Verification items for the finished model (mm, model axes). A direction names the side the tool comes from. Round coordinates to 2 decimals unless told otherwise and drop trailing zeros. Order: outer loops, then holes, each group sorted by start corner. A loop starts at its lowest first (then second) coordinate and runs counter-clockwise, first axis right, second up. Notation, with made-up numbers: (75, -33) -> (79, -33) arc R22 ccw to (79, 0) -> close; hole circle Ø9 at (-5.75, -23). An arc over 180 degrees is marked (long way). Put each result on its own line as item: value.
from build123d import *

# Parameters (mm, degrees)
BOSS_EXTRUDE1_DEPTH = 26
SKETCH3_R           = 2.25
CUT_EXTRUDE1_DEPTH  = 50.759421218
SKETCH2_R           = 2.5
CUT_EXTRUDE2_DEPTH  = 50.759421218
SKETCH4_R           = 5
CUT_EXTRUDE3_DEPTH  = 45.452221542
SKETCH5_R           = 4
CUT_EXTRUDE4_DEPTH  = 45.452221542
CHAMFER1_SIZE       = 3
FILLET2_R           = 4


with BuildPart() as part:
    # Sketch1 → Boss-Extrude1 (new body)
    with BuildSketch(Plane.XY):
        Polygon((0, 0), (10, 0), (30, 20), (30, 30), (0, 30), align=None)
    extrude(amount=BOSS_EXTRUDE1_DEPTH)

    # Sketch3 → Cut-Extrude1 (cut, through all)
    with BuildSketch(Plane(origin=(0, 30, 0), x_dir=(1, 0, 0), z_dir=(0, 1, 0))):
        with Locations(Location((20, -6, 0), (0, 0, 180))):
            Circle(SKETCH3_R)
    extrude(amount=-CUT_EXTRUDE1_DEPTH, mode=Mode.SUBTRACT)

    # Sketch2 → Cut-Extrude2 (cut, through all)
    with BuildSketch(Plane.ZY):
        with Locations(Location((18, 10, 0), (0, 0, 270))):
            Circle(SKETCH2_R)
    extrude(amount=-CUT_EXTRUDE2_DEPTH, mode=Mode.SUBTRACT)

    # Sketch4 → Cut-Extrude3 (cut, through all)
    with BuildSketch(Plane.ZY.offset(-10)):
        with Locations(Location((18, 10, 0), (0, 0, 270))):
            Circle(SKETCH4_R)
    extrude(amount=-CUT_EXTRUDE3_DEPTH, mode=Mode.SUBTRACT)

    # Sketch5 → Cut-Extrude4 (cut, through all)
    with BuildSketch(Plane(origin=(0, 20, 0), x_dir=(1, 0, 0), z_dir=(0, 1, 0))):
        with Locations(Location((20, -6, 0), (0, 0, 180))):
            Circle(SKETCH5_R)
    extrude(amount=-CUT_EXTRUDE4_DEPTH, mode=Mode.SUBTRACT)

    # Chamfer1
    # the kernel refuses this chamfer: 3 mm, written as the material it adds along each edge
    with BuildSketch(Plane(origin=(10, 10, 18), x_dir=(0, -1, 0), z_dir=(0, 0, -1))) as chamfer1_piece_1_section:
        Polygon((5, -CHAMFER1_SIZE), (5 - CHAMFER1_SIZE, 0), (5, 0), align=None)
    chamfer1_piece_1 = revolve(axis=Axis((10, 10, 18), (-1, 0, 0)), mode=Mode.PRIVATE)
    chamfer1_piece_1 = chamfer1_piece_1 - Plane(origin=(11.757355127, 10, 18), x_dir=(0, -1, 0), z_dir=(-1, 0, 0)) * Cylinder(2.5, 20, mode=Mode.PRIVATE)
    add(chamfer1_piece_1)

    # Fillet2
    fillet2_edges = [part.edges().sort_by_distance(p)[0] for p in [
        (30, 20, 13),
        (10, 0, 13),
    ]]
    fillet(fillet2_edges, radius=FILLET2_R)


solid = part.part
Item 1: Tool access check on faces 4 (the cylindrical face through (16.185, 14.654, 7.201)), 5 (the cylindrical face through (9.89, 0.31, 13.18)). Record the directions out of +Z, -Z, +X, -X, +Y, -Y that give a thin tool (end or side, any length) a straight path to the whole face; none if there is none.
Check sheet entries:
face 4: -Y
face 5: +Z, -Z, +X, -Y
Item 2: Material ranges on L1, parallel to Z at x = 20, y = 12.75; L2, parallel to Z at x = 4, y = 11.5; L3, parallel to Z at x = 20, y = 22.25, recorded low to high. Write a range as [from, to].
Check sheet entries:
L1: z = [0, 2], [10, 13.82], [22.18, 26]
L2: z = [0, 16], [20, 26]
L3: z = [0, 3.75], [8.25, 26]
Item 3: Release check for a two-part mould opening along Y. For faces 1 (the cylindrical face through (18, 15, 18)), 2 (the cylindrical face through (29.69, 20.11, 13.18)), 3 (the flat face through (30, 26, 13)) record: +Y half, -Y half, draft (parallel to the pull), parting line (faces both ways), or undercut.
Check sheet entries:
face 1: undercut
face 2: -Y half
face 3: draft
Item 4: Section check A-A on z = 6. Record the boundary of the cut face in (x, y).
Check sheet entries:
outline: (0, 0) -> (8.34, 0) arc R4 ccw to (11.17, 1.17) -> (16, 6) -> (16, 20) -> (17.75, 20) -> (17.75, 30) -> (0, 30) -> close; (22.25, 20) -> (24, 20) -> (24, 14) -> (28.83, 18.83) arc R4 ccw to (30, 21.66) -> (30, 30) -> (22.25, 30) -> close
Item 5: Section check C-C on y = 10. Record the boundary of the cut face in (x, z).
Check sheet entries:
outline: (0, 0) -> (20, 0) -> (20, 2) arc R4 cw to (20, 10) -> (20, 13) -> (13, 13) -> (10.5, 15.5) -> (0, 15.5) -> close; (0, 20.5) -> (10.5, 20.5) -> (13, 23) -> (20, 23) -> (20, 26) -> (0, 26) -> close
Item 6: Gauge pin test, flat ends, axial feed: pin 1 Ø4 at (x, z) = (26.5, 17) entering from -Y; pin 2 Ø7 at (x, z) = (20, 6) entering from -Y; pin 3 Ø9 at (x, z) = (20, 6) entering from -Y; pin 4 Ø4 at (y, z) = (10, 18) entering from -X (3 decimals). Record the tip position at first contact, or that the pin passes through.
Check sheet entries:
pin 1: stops at y = 14.67
pin 2: stops at y = 20
pin 3: stops at y = 5.5
pin 4: passes through
Item 7: Section check D-D on y = 18. Record the boundary of the cut face in (x, z).
Check sheet entries:
outline: (0, 0) -> (28, 0) -> (28, 26) -> (0, 26) -> close; hole circle Ø8 at (20, 6)
Item 8: Section check B-B on x = 20. Record the boundary of the cut face in (y, z), then the cut area to 3 significant figures.
Check sheet entries:
outline: (10, 0) -> (30, 0) -> (30, 3.75) -> (20, 3.75) -> (20, 2) -> (10, 2) -> close; (10, 10) -> (20, 10) -> (20, 8.25) -> (30, 8.25) -> (30, 26) -> (10, 26) -> (10, 23) arc R5 cw to (10, 13) -> close
area: 356 mm^2
